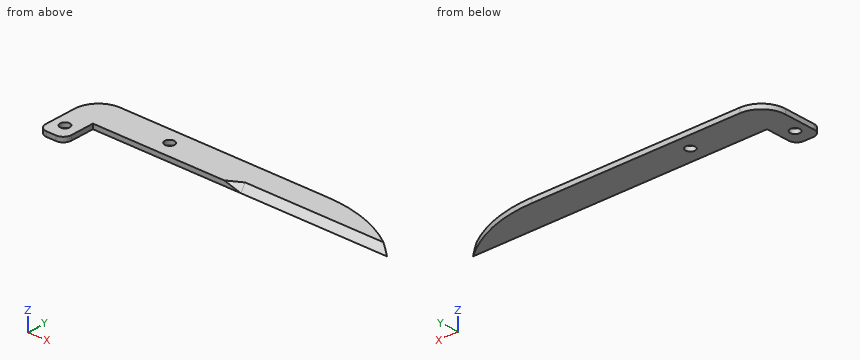
```python
from build123d import *

# Parameters (mm, degrees)
SKETCH_1_W          = 200
SKETCH_1_H          = 20
EXTRUDE_1_DEPTH     = 3
CUT_EXTRUDE_1_REACH = 202.272
CHAMFER_1_SIZE      = 4
CHAMFER_1_SIZE_2    = 6.92820323
CUT_EXTRUDE_2_DEPTH = 101.543522914
SKETCH_5_R          = 3
CUT_EXTRUDE_3_DEPTH = 4
SKETCH_8_W          = 16
SKETCH_8_H          = 20
EXTRUDE_2_DEPTH     = 3
SKETCH_7_R          = 3
CUT_EXTRUDE_5_DEPTH = 10
FILLET_1_R          = 15
FILLET_2_R          = 5


with BuildPart() as part:
    # 草图1 → 凸台-拉伸1 (new body)
    with BuildSketch(Plane.XY):
        Rectangle(SKETCH_1_W, SKETCH_1_H)
    extrude(amount=EXTRUDE_1_DEPTH)

    # 切除-拉伸1: up to this plane
    cut_extrude_1_end = Plane(origin=(7.330127019, -12.696152423, 0), z_dir=(-0.49999999999999445, 0.8660254037844419, 0))
    # 草图3 → 切除-拉伸1 (cut, up to the surface)
    with BuildSketch(Plane(origin=(100, 0, 0), x_dir=(0, 0, -1), z_dir=(1, 0, 0)), mode=Mode.PRIVATE) as cut_extrude_1_sk1:
        Polygon((-3, -5), (0, -10), (-3, -10), align=None)
    cut_extrude_1_tool1 = split(extrude(cut_extrude_1_sk1.sketch, amount=-CUT_EXTRUDE_1_REACH, mode=Mode.PRIVATE), bisect_by=cut_extrude_1_end, keep=Keep.BOTH, mode=Mode.PRIVATE)
    add(cut_extrude_1_tool1.solids().sort_by_distance((100, -8.333333, 2))[0], mode=Mode.SUBTRACT)

    # 倒角1
    # the kernel refuses this chamfer: 6.92820323, 4 mm, written as the material it takes off along each edge
    with BuildSketch(Plane(origin=(-3.522514528, -18.961927941, 3), x_dir=(0.02894693120133512, -0.05013755556391397, -0.9983227437537926), z_dir=(0.8660254037844419, 0.49999999999999445, 0))) as chamfer_1_piece_1_section:
        Polygon((CHAMFER_1_SIZE * 0.998322743754, CHAMFER_1_SIZE * 0.0578938624027), (-CHAMFER_1_SIZE_2 * 0.057893862405, CHAMFER_1_SIZE_2 * 0.998322743793), (0, 0), align=None)
    chamfer_1_piece_1 = extrude(amount=45.847711765, mode=Mode.PRIVATE)
    chamfer_1_piece_1 = split(chamfer_1_piece_1, bisect_by=Plane(origin=(9.642486401, -7.716503268, 1.370098039), z_dir=(0, -0.5144957554275265, 0.8574929257125443)), keep=Keep.TOP, mode=Mode.PRIVATE)
    add(chamfer_1_piece_1, mode=Mode.SUBTRACT)

    # 草图4 → 切除-拉伸2 (cut, through all)
    with BuildSketch(Plane.XY.offset(3)):
        with BuildLine():
            Line((45, 10), (45, 14.118329336))
            Line((45, 14.118329336), (100, 14.118329336))
            Line((100, 14.118329336), (100, -10))
            add(Edge.make_bspline(
                [(100, -10), (75.292472647, 10), (45, 10)],
                knots=[0, 0, 0, 1, 1, 1], degree=2))
        make_face()
    extrude(amount=-CUT_EXTRUDE_2_DEPTH, mode=Mode.SUBTRACT)

    # 草图5 → 切除-拉伸3 (cut)
    with BuildSketch(Plane.XY.offset(3)):
        with Locations((-45, 0)):
            Circle(SKETCH_5_R)
    extrude(amount=-CUT_EXTRUDE_3_DEPTH, mode=Mode.SUBTRACT)

    # 草图8 → 凸台-拉伸2 (add)
    with BuildSketch(Plane.XY.offset(3)):
        with Locations((-92, -20)):
            Rectangle(SKETCH_8_W, SKETCH_8_H)
    extrude(amount=-EXTRUDE_2_DEPTH)

    # 草图7 → 切除-拉伸5 (cut)
    with BuildSketch(Plane.XY.offset(3)):
        with Locations((-92.5, -20)):
            Circle(SKETCH_7_R)
    extrude(amount=-CUT_EXTRUDE_5_DEPTH, mode=Mode.SUBTRACT)

    # 圆角1
    fillet_1_edges = [part.edges().sort_by_distance(p)[0] for p in [
        (-100, 10, 1.5),
    ]]
    fillet(fillet_1_edges, radius=FILLET_1_R)

    # 圆角2
    fillet_2_edges = [part.edges().sort_by_distance(p)[0] for p in [
        (-84, -30, 1.5),
        (-100, -30, 1.5),
    ]]
    fillet(fillet_2_edges, radius=FILLET_2_R)


solid = part.part
```
Design review of the part built by this model. Coordinates are the model's own, in mm. Round coordinates to 2 decimals unless told otherwise and drop trailing zeros. Order: outer loops, then holes, each group sorted by start corner. A loop starts at its lowest first (then second) coordinate and runs counter-clockwise, first axis right, second up. Notation, with made-up numbers: (32, -2.75) - (45, -2.75) arc R16 ccw to (45, 12.25) - close; hole circle Ø2 at (57, 1.5). An arc over 180 degrees is marked (long way). Return JSON: item names as keys, results as strings.
Q1. Consider section C-C on z = 1.8. Give the number of separate pieces and of enclosed holes in the cut face, plus the area to 3 significant figures.
Computed values:
{"separate pieces": "1", "enclosed holes": "2", "area": "3,580 mm2"}
Q2. Wall thickness on L1, parallel to Y at x = -45, z = 2.1; L2, parallel to Y at x = -92.5, z = 1.7; L3, parallel to X at y = -17.5, z = 1.4: over which ranges is each line inside the solid? List them lowest first. Write a range as [from, to].
Computed values:
{"L1": "y = [-10, -3], [3, 10]", "L2": "y = [-30, -23], [-17, 7.99]", "L3": "x = [-100, -94.16], [-90.84, -84]"}
Q3. For pin 1 Ø1.5 at (y, z) = (-3.5, 1) entering from -X; pin 2 Ø0.9 at (x, z) = (-31, 1.5) entering from -Y; pin 3 Ø1.5 at (y, z) = (4.5, 2.5) entering from +X, all flat-tipped, find the tip position at first contact; note any pin that passes through.
Computed values:
{"pin 1": "stops at x = -99.98", "pin 2": "stops at y = -10", "pin 3": "stops at x = 77.12"}
Q4. Consider section A-A on y = -20. Write out the cut boundary in (x, z), plus the area to 3 significant figures.
Computed values:
{"outline": "(-100, 0) - (-95.5, 0) - (-95.5, 3) - (-100, 3) - close; (-89.5, 0) - (-84, 0) - (-84, 3) - (-89.5, 3) - close", "area": "30.0 mm2"}
Q5. Consider section D-D on x = 39.5. Write out the cut boundary in (y, z).
Computed values:
{"outline": "(-10, 0) - (10, 0) - (10, 3) - (-5, 3) - close"}
Q6. Consider section B-B on x = -45. Write out the cut boundary in (y, z).
Computed values:
{"outline": "(-10, 0) - (-3, 0) - (-3, 3) - (-10, 3) - close; (3, 0) - (10, 0) - (10, 3) - (3, 3) - close"}
